from build123d import *

# Parameters (mm, degrees)
SALIENTE_EXTRUIR1_DEPTH = 17
CROQUIS2_W              = 100
CROQUIS2_H              = 12.5
CORTAR_EXTRUIR1_DEPTH   = 8
CROQUIS3_R              = 3
CORTAR_EXTRUIR2_DEPTH   = 17


with BuildPart() as part:
    # Croquis1 → Saliente-Extruir1 (new body)
    with BuildSketch(Plane(origin=(0, 0, 0), x_dir=(1, 0, 0), z_dir=(0, 1, 0))):
        Polygon((0, 0), (-20, 0), (-20, 80), (80, 80), (80, 0), (60, 0), (60, 65), (0, 65), align=None)
    extrude(amount=SALIENTE_EXTRUIR1_DEPTH)

    # Croquis2 → Cortar-Extruir1 (cut)
    with BuildSketch(Plane.XY):
        with Locations((30, 8.5)):
            Rectangle(CROQUIS2_W, CROQUIS2_H)
    extrude(amount=-CORTAR_EXTRUIR1_DEPTH, mode=Mode.SUBTRACT)

    # Croquis3 → Cortar-Extruir2 (cut)
    with BuildSketch(Plane(origin=(0, 17, 0), x_dir=(1, 0, 0), z_dir=(0, 1, 0))):
        with Locations(Location((-10, 15, 0), (0, 0, 270))):
            Circle(CROQUIS3_R)
        with Locations(Location((70, 15, 0), (0, 0, 270))):
            Circle(CROQUIS3_R)
    extrude(amount=-CORTAR_EXTRUIR2_DEPTH, mode=Mode.SUBTRACT)


solid = part.part
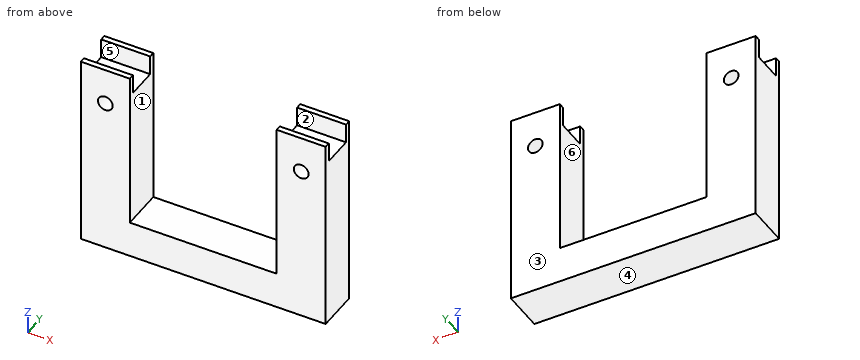
Could you check a few things on this model? Use its own coordinates, in mm. Face numbers are marked on the shaded views. A direction names the side the tool comes from. Give positions to 0.01 mm unless a question says otherwise; leave off trailing zeros. Write each loop counter-clockwise with the first axis right and the second up, starting at its lowest first coordinate (ties: lowest second). Pieces come first, ordered by that corner, then holes. Notation, with made-up numbers: (-21, 78.25) -> (9, 78.25) arc R13 ccw to (9, 95.25) -> close; hole circle Ø9 at (27, 77). An arc over 180 degrees is marked (long way). Write each question's results on one line, items separated by ' | '. Start each with the question number.
Q1. Suppose I cut it at C-C, the plane z = -15. List the corners of the cut face in (x, y) for me, and give its area (3 significant figures).
Q2. I need wall thicknesses on probe 1 along X at (y, z) = (9.25, -15); probe 2 along X at (y, z) = (10, -54); probe 3 along Z at (x, y) = (14, 13.25). Which ranges of each line are inside material? Lowest first, please.
Q3. We'd pull the mould along Y, two halves only. Please class the marked faces 1, 2 and 3: +Y half, -Y half, draft (parallel to the pull), parting line (faces both ways), or undercut.
Q4. I'm going to push flat-ended pins straight in: pin 1 Ø6 at (x, y) = (75, 7) entering from +Z; pin 2 Ø5.5 at (x, z) = (70, -15) entering from +Y. Where does each tip first touch, or does it pass through?
Q5. Which directions (+Z, -Z, +X, -X, +Y, -Y) give clear straight access to the entire face, cutting with the end or side of a thin tool? Please do the marked faces 4, 5 and 6.
Q6. Suppose I cut it at A-A, the plane x = -10. List the corners of the cut face in (y, z) for me.
Q7. Suppose I cut it at B-B, the plane z = -47. List the corners of the cut face in (x, y) for me.
Q8. Suppose I cut it at D-D, the plane x = 63.5. List the corners of the cut face in (y, z) for me.
Outcome:
1) outline: (-20, 0) -> (-13, 0) -> (-13, 17) -> (-20, 17) -> close; (-7, 0) -> (0, 0) -> (0, 17) -> (-7, 17) -> close; (60, 0) -> (67, 0) -> (67, 17) -> (60, 17) -> close; (73, 0) -> (80, 0) -> (80, 17) -> (73, 17) -> close | area: 476 mm2
2) probe 1: -20 to -13, -7 to 0, 60 to 67, 73 to 80 | probe 2: -20 to 0, 60 to 80 | probe 3: -80 to -65
3) face 1: draft | face 2: undercut | face 3: +Y half
4) pin 1: z = -8 | pin 2: through
5) face 4: -Z, +X, -X, +Y, -Y | face 5: +Z, +X, -X | face 6: +Z, +Y, -Y
6) outline: (0, -80) -> (17, -80) -> (17, -18) -> (0, -18) -> close; (0, -12) -> (17, -12) -> (17, 0) -> (14.75, 0) -> (14.75, -8) -> (2.25, -8) -> (2.25, 0) -> (0, 0) -> close
7) outline: (-20, 0) -> (0, 0) -> (0, 17) -> (-20, 17) -> close; (60, 0) -> (80, 0) -> (80, 17) -> (60, 17) -> close
8) outline: (0, -80) -> (17, -80) -> (17, 0) -> (14.75, 0) -> (14.75, -8) -> (2.25, -8) -> (2.25, 0) -> (0, 0) -> close
